Read the model definition and answer for the solid it produces. Units are mm, in the model's axes. Face numbers are marked on the shaded views. Coordinates: 2 decimals unless noted, no trailing zeros. Order: outer loops, then holes, each group sorted by start corner. A loop starts at its lowest first (then second) coordinate and runs counter-clockwise, first axis right, second up. Notation, with made-up numbers: M -4.5,85 L 18.5,85 A26 cw 18.5,115 Z; hole C 6.5,43.5 d7. An arc over 180 degrees is marked long. One line per question, with ' | ' between items. Start each with the question number.
1) Consider probe 1 along X at (y, z) = (-18, -26); probe 2 along Z at (x, y) = (0, -29); probe 3 along Z at (x, y) = (-6.5, -2). Determine where each line is inside the solid, lowest interval first.
2) Find section C-C, the plane x = 16. Write down the section's boundary in (y, z).
3) Find section A-A, the plane z = -20. Write down the section's boundary in (x, y), plus the area to 3 significant figures.
4) The mould has two halves that part along X. Classify the marked faces 1, 2, 3 and 4: +X half, -X half, draft (parallel to the pull), parting line (faces both ways), or undercut.
5) Find section B-B, the plane y = -15. Write down the section's boundary in (x, z), plus the area to 3 significant figures.
6) Find section D-D, the plane x = 0. Write down the section's boundary in (y, z), plus the area to 3 significant figures.
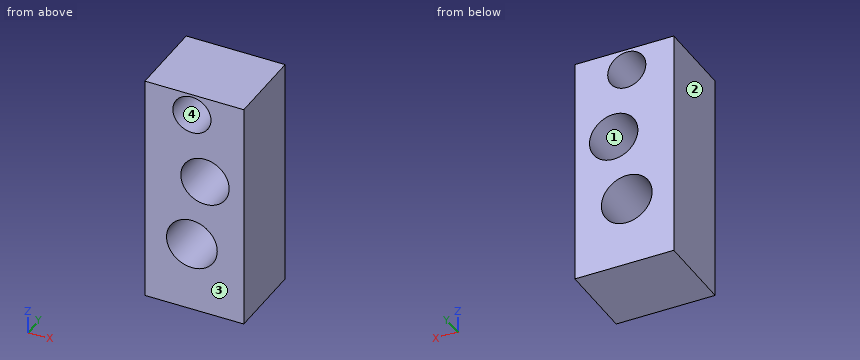
from build123d import *

# Parameters (mm, degrees)
F0_W     = 51.029243
F0_H     = 118.811481
F0_R     = 13.085796
F0_R_2   = 9.837697
F0_R_3   = 12.472461
F1_DEPTH = 41.402
F2_DEPTH = 25.4


with BuildPart() as f1:
    # F0 (on Front) → F1 (new body)
    with BuildSketch(Plane.XZ):
        with Locations((1.25166, -2.695885)):
            Rectangle(F0_W, F0_H)
        with Locations((0, -26.09231)):
            Circle(F0_R, mode=Mode.SUBTRACT)
        with Locations((0, 45.54119)):
            Circle(F0_R_2, mode=Mode.SUBTRACT)
        with Locations((6.739711, 10.494693)):
            Circle(F0_R_3, mode=Mode.SUBTRACT)
    extrude(amount=F1_DEPTH)

    # F0 (on Front) → F2 (join)
    with BuildSketch(Plane.XZ):
        with Locations((1.25166, -2.695885)):
            Rectangle(F0_W, F0_H)
        with Locations((0, -26.09231)):
            Circle(F0_R, mode=Mode.SUBTRACT)
        with Locations((0, 45.54119)):
            Circle(F0_R_2, mode=Mode.SUBTRACT)
        with Locations((6.739711, 10.494693)):
            Circle(F0_R_3, mode=Mode.SUBTRACT)
    extrude(amount=F2_DEPTH)


solid = f1.part
Report:
1) probe 1: x = -24.26 to -13.09, 13.09 to 26.77 | probe 2: z = -62.1 to -39.18, -13.01 to 0, 20.99 to 35.7, 55.38 to 56.71 | probe 3: z = -62.1 to -37.45, -14.74 to 38.16, 52.93 to 56.71
2) outline: M -41.4,-62.1 L 0,-62.1 L 0,2.14 L -41.4,2.14 Z; M -41.4,18.85 L 0,18.85 L 0,56.71 L -41.4,56.71 Z
3) outline: M -24.26,-41.4 L -11.58,-41.4 L -11.58,0 L -24.26,0 Z; M 11.58,-41.4 L 26.77,-41.4 L 26.77,0 L 11.58,0 Z | area: 1,150 mm^2
4) face 1: undercut | face 2: -X half | face 3: draft | face 4: undercut
5) outline: M -24.26,-62.1 L 26.77,-62.1 L 26.77,56.71 L -24.26,56.71 Z; hole C 0,-26.09 d26.17; hole C 0,45.54 d19.68; hole C 6.74,10.49 d24.94 | area: 4,730 mm^2
6) outline: M -41.4,-62.1 L 0,-62.1 L 0,-39.18 L -41.4,-39.18 Z; M -41.4,-13.01 L 0,-13.01 L 0,0 L -41.4,0 Z; M -41.4,20.99 L 0,20.99 L 0,35.7 L -41.4,35.7 Z; M -41.4,55.38 L 0,55.38 L 0,56.71 L -41.4,56.71 Z | area: 2,150 mm^2
